```python
from build123d import *

# Parameters (mm, degrees)
F0_R         = 3
F1_DEPTH     = 25
F3_DEPTH     = 18.001
F4_T1_DEPTH  = 25
F4_T3_DEPTH  = 25
F4_T5_DEPTH  = 25
F4_T7_DEPTH  = 25
F4_T9_DEPTH  = 35
F4_T11_DEPTH = 30.1931758285
F4_T13_DEPTH = 30.1931758285
F4_T15_DEPTH = 35


# Not quite as in the source:
# - a fillet or chamfer that OpenCascade refuses, or shapes differently, is made with other operations: its cross-section is extruded or revolved along the edge and cut away or added


with BuildPart() as f1:
    # F0 (on Front) → F1 (new body)
    with BuildSketch(Plane.XZ):
        Polygon((15, 9), (-15, 9), (-15, 3), (-14, 3), (-14, -6), (-7, -6), (-4.890570417, -9), (4.890570417, -9), (7, -6), (14, -6), (14, 3), (15, 3), align=None)
        Circle(F0_R, mode=Mode.SUBTRACT)
    extrude(amount=F1_DEPTH)

    # F2 (on face) → F3 (cut, through all)
    with BuildSketch(Plane.XY.offset(9)):
        with BuildLine():
            Line((10, -5), (10, -6))
            ThreePointArc((10, -6), (10.7071067812, -5.7071067812), (11, -5))
            ThreePointArc((11, -5), (10, -4), (9, -5))
            Line((9, -5), (10, -5))
        make_face()
        with BuildLine():
            ThreePointArc((9, -5), (9.2928932188, -5.7071067812), (10, -6))
            Line((10, -6), (10, -5))
            Line((10, -5), (9, -5))
        make_face()
        with BuildLine():
            Line((10, -20), (9, -20))
            ThreePointArc((9, -20), (10, -21), (11, -20))
            ThreePointArc((11, -20), (10.7071067812, -19.2928932188), (10, -19))
            Line((10, -19), (10, -20))
        make_face()
        with BuildLine():
            ThreePointArc((10, -19), (9.2928932188, -19.2928932188), (9, -20))
            Line((9, -20), (10, -20))
            Line((10, -20), (10, -19))
        make_face()
        with BuildLine():
            ThreePointArc((-10, -19), (-10.7071067812, -20.7071067812), (-9, -20))
            Line((-9, -20), (-10, -20))
            Line((-10, -20), (-10, -19))
        make_face()
        with BuildLine():
            Line((-10, -20), (-9, -20))
            ThreePointArc((-9, -20), (-9.2928932188, -19.2928932188), (-10, -19))
            Line((-10, -19), (-10, -20))
        make_face()
        with BuildLine():
            ThreePointArc((-9, -5), (-10.7071067812, -4.2928932188), (-10, -6))
            Line((-10, -6), (-10, -5))
            Line((-10, -5), (-9, -5))
        make_face()
        with BuildLine():
            Line((-10, -5), (-10, -6))
            ThreePointArc((-10, -6), (-9.2928932188, -5.7071067812), (-9, -5))
            Line((-9, -5), (-10, -5))
        make_face()
    extrude(amount=-F3_DEPTH, mode=Mode.SUBTRACT)

    # F4: fillet of radius 2 on 8 edges, made by hand

    # F4_s2 → F4_t1 (join)
    with BuildSketch(Plane.XZ):
        with BuildLine():
            ThreePointArc((15, 3), (14.2679491924, 2.2679491924), (14, 1.2679491924))
            Line((14, 1.2679491924), (14, 3))
            Line((14, 3), (15, 3))
        make_face()
    extrude(amount=F4_T1_DEPTH)

    # F4_s4 → F4_t3 (join)
    with BuildSketch(Plane.XZ):
        with BuildLine():
            ThreePointArc((-15, 3), (-14.2679491924, 2.2679491924), (-14, 1.2679491924))
            Line((-14, 1.2679491924), (-14, 3))
            Line((-14, 3), (-15, 3))
        make_face()
    extrude(amount=F4_T3_DEPTH)

    # F4_s6 → F4_t5 (join)
    with BuildSketch(Plane.XZ):
        with BuildLine():
            ThreePointArc((-8.0386351657, -6), (-7.1168832592, -6.2250708682), (-6.4025908546, -6.8496265771))
            Line((-6.4025908546, -6.8496265771), (-7, -6))
            Line((-7, -6), (-8.0386351657, -6))
        make_face()
    extrude(amount=F4_T5_DEPTH)

    # F4_s8 → F4_t7 (join)
    with BuildSketch(Plane.XZ):
        with BuildLine():
            ThreePointArc((6.4025908546, -6.8496265771), (7.1168832592, -6.2250708682), (8.0386351657, -6))
            Line((8.0386351657, -6), (7, -6))
            Line((7, -6), (6.4025908546, -6.8496265771))
        make_face()
    extrude(amount=F4_T7_DEPTH)

    # F4_s10 → F4_t9 (cut)
    with BuildSketch(Plane.XZ.offset(-5)):
        with BuildLine():
            ThreePointArc((-14, -4), (-13.4142135624, -5.4142135624), (-12, -6))
            Line((-12, -6), (-14, -6))
            Line((-14, -6), (-14, -4))
        make_face()
    extrude(amount=F4_T9_DEPTH, mode=Mode.SUBTRACT)

    # F4_s12 → F4_t11 (cut)
    with BuildSketch(Plane.XZ.offset(-2.5965879143)):
        with BuildLine():
            ThreePointArc((-3.8519352513, -9), (-4.7736871578, -8.7749291318), (-5.4879795624, -8.1503734229))
            Line((-5.4879795624, -8.1503734229), (-4.890570417, -9))
            Line((-4.890570417, -9), (-3.8519352513, -9))
        make_face()
    extrude(amount=F4_T11_DEPTH, mode=Mode.SUBTRACT)

    # F4_s14 → F4_t13 (cut)
    with BuildSketch(Plane.XZ.offset(-2.5965879143)):
        with BuildLine():
            ThreePointArc((5.4879795624, -8.1503734229), (4.7736871578, -8.7749291318), (3.8519352513, -9))
            Line((3.8519352513, -9), (4.890570417, -9))
            Line((4.890570417, -9), (5.4879795624, -8.1503734229))
        make_face()
    extrude(amount=F4_T13_DEPTH, mode=Mode.SUBTRACT)

    # F4_s16 → F4_t15 (cut)
    with BuildSketch(Plane.XZ.offset(-5)):
        with BuildLine():
            ThreePointArc((14, -4), (13.4142135624, -5.4142135624), (12, -6))
            Line((12, -6), (14, -6))
            Line((14, -6), (14, -4))
        make_face()
    extrude(amount=F4_T15_DEPTH, mode=Mode.SUBTRACT)


solid = f1.part
```
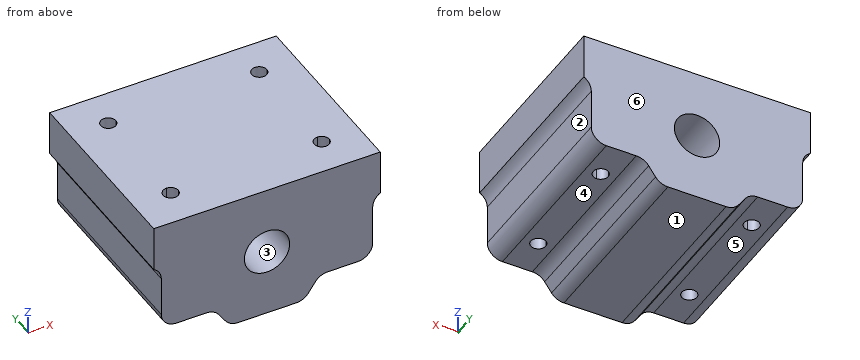
Build history of the part. All positions in model axes, mm. Face numbers are marked on the shaded views. A direction names the side the tool comes from. Round coordinates to 2 decimals unless told otherwise and drop trailing zeros. Loops run counter-clockwise (first coordinate to the right, second up) from the corner with the lowest first, then second, coordinate; pieces in that order, holes last.
Item 1: Two-plate mould, pull along X, no slides. Class the marked faces 1, 2 and 3: released by +X, released by -X, zero draft, split by the parting line, or undercut.
Item 2: Drill centre lines: line 1 along Y through (x, z) = (-10, -0.25); line 2 along X through (y, z) = (-19.75, 5.5); line 3 along X through (y, z) = (-20, 0.75). Where is each one in solid material? Low to high.
Item 3: Saw through at C-C (y = -9.25). List the corners of the cut face in (x, z).
Item 4: Saw through at A-A (z = 3.5). List the corners of the cut face in (x, y), then the cut area to 3 significant figures.
Item 5: Pin check, flat tips, straight feed: P1, Ø1.6, axis at y = -18, z = -1, coming from the -X side; P2, Ø6, axis at x = -11.5, y = -7.5, coming from the -Z side; P3, Ø2.5, axis at y = -17, z = -0.5, coming from the +X side. Stop position of each tip, or through.
Item 6: Saw through at B-B (x = 0). List the corners of the cut face in (y, z).
Item 7: Which spindle directions (+Z, -Z, +X, -X, +Y, -Y) get a long thin tool onto all of the face, cutting with end or side? Do the marked faces 4, 5 and 6. Say none if no direction does.
Item 8: Saw through at D-D (z = -0.75). List the corners of the cut face in (x, y).
Worked answers:
1. face 1: zero draft
1. face 2: released by +X
1. face 3: undercut
2. line 1: y = -25 to -21, -19 to -6, -4 to 0
2. line 2: x = -15 to -10.97, -9.03 to 9.03, 10.97 to 15
2. line 3: x = -14 to -11, -9 to -2.9, 2.9 to 9, 11 to 14
3. outline: (-15, 3) arc R2 cw to (-14, 1.27) - (-14, -4) arc R2 ccw to (-12, -6) - (-8.04, -6) arc R2 cw to (-6.4, -6.85) - (-5.49, -8.15) arc R2 ccw to (-3.85, -9) - (3.85, -9) arc R2 ccw to (5.49, -8.15) - (6.4, -6.85) arc R2 cw to (8.04, -6) - (12, -6) arc R2 ccw to (14, -4) - (14, 1.27) arc R2 cw to (15, 3) - (15, 9) - (-15, 9) - close; hole circle Ø6 at (0, 0)
4. outline: (-15, -25) - (15, -25) - (15, 0) - (-15, 0) - close; hole circle Ø2 at (-10, -20); hole circle Ø2 at (-10, -5); hole circle Ø2 at (10, -20); hole circle Ø2 at (10, -5)
4. area: 737 mm2
5. P1: stops at x = -14
5. P2: stops at z = -6
5. P3: stops at x = 14
6. outline: (-25, -9) - (0, -9) - (0, -3) - (-25, -3) - close; (-25, 3) - (0, 3) - (0, 9) - (-25, 9) - close
7. face 4: -Z, +X, +Y, -Y
7. face 5: -Z, -X, +Y, -Y
7. face 6: +Z, -Z, +X, -X, +Y
8. outline: (-14, -25) - (-2.9, -25) - (-2.9, 0) - (-14, 0) - close; (2.9, -25) - (14, -25) - (14, 0) - (2.9, 0) - close; hole circle Ø2 at (-10, -20); hole circle Ø2 at (-10, -5); hole circle Ø2 at (10, -20); hole circle Ø2 at (10, -5)
